Autodesk Inventor part; units mm, degrees
ref_plane "YZ Plane" through (0, 0, 0) normal (1, 0, 0) x (0, 1, 0)
ref_plane "XZ Plane" through (0, 0, 0) normal (0, 1, 0) x (-1, 0, 0)
ref_plane "XY Plane" through (0, 0, 0) normal (0, 0, 1) x (1, 0, 0)
sketch "Sketch1" plane through (0, 0, 0) normal (0, 0, 1) x (1, 0, 0)
  circle A0 centre (0, 0) radius 4
  dimension "d0" = 8
extrude "Extrusion1" add sketch "Sketch1" along normal blind 15
sketch "Sketch2" plane through (0, 0, 15) normal (0, 0, 1) x (1, 0, 0)
  circle A0 centre (0, 0) radius 4
  line L0 (0, -5.6) -> (0, 5.6)
  line L1 (1.5, -3.7081) -> (1.5, 3.7081)
  line L2 (-1.5, -3.7081) -> (-1.5, 3.7081)
  circle A1 centre (0, 0) radius 4
  dimension "d5" = 3
  dimension "d6" = 1.5
extrude "Extrusion2" cut sketch "Sketch2" against normal blind 3 contours L1 A0 L0 | L0 A0 L2
fillet "Fillet1" radius 0.5 14 edges at (-1.5, 0, 15) (1.5, 0, 15) (-1.5, 0, 12) (1.5, 0, 12) (3.3166, -2.2361, 15) (3.3166, 2.2361, 15) (-4, 0, 15) (-1.5, -3.7081, 13.5) (-1.5, 3.7081, 13.5) (1.5, -3.7081, 13.5) (1.5, 3.7081, 13.5) (0, -4, 12) (0, 4, 12) (-4, 0, 0)
properties part number "Locating Pin"
For this review, take the finished solid that the model builds, in its own axes (mm). A direction names the side the tool comes from. Round coordinates to 2 decimals unless told otherwise and drop trailing zeros. Write each loop counter-clockwise with the first axis right and the second up, starting at its lowest first coordinate (ties: lowest second). Pieces come first, ordered by that corner, then holes. Notation, with made-up numbers: M 3.5,-10.5 L 25.5,-10.5 A35 cw 25.5,24.5 Z; hole C 37.25,17 d6. An arc over 180 degrees is marked long. Write item = value, one per line. Start each with the question number.
(1) Clearance check with flat-ended pins moving along their axes: pin 1 Ø0.6 at (x, y) = (0, 1.5) entering from +Z; pin 2 Ø1.5 at (y, z) = (1.5, 11) entering from -X; pin 3 Ø1.5 at (y, z) = (3, 5) entering from -X. State where each tip first meets the part, or that it passes through.
(2) We need section A-A (z = 13). Give the boundary of the cut face in (x, y), then the cut area to 3 significant figures.
(3) The part is to be moulded in two halves that separate along X. For faces 1 (the face through (0, 0, 12)), 2 (the face through (-4, 0, 7)), 3 (the face through (0, 0, 0)), say which applies: +X half, -X half, draft (parallel to the pull), parting line (faces both ways), or undercut.
(4) For faces 4 (the face through (-3, 0, 15)), 5 (the face through (1.5, 0, 14)), list the 3-axis set-ups (+Z, -Z, +X, -X, +Y, -Y) from which the entire face can be reached by the end or side of a thin tool; tool diameter is ignored.
(5) We need section D-D (z = 6.25). Give the boundary of the cut face in (x, y).
(6) We need section B-B (x = 0). Give the boundary of the cut face in (y, z).
(7) For line 1 along Z through (x, y) = (0, 1.25); line 2 along Z through (x, y) = (3.5, 0.5); line 3 along Y through (x, z) = (2.75, 1.25), list the stretches that pass through material, from the lowest coordinate up.
(8) We need section C-C (y = 0). Give the boundary of the cut face in (x, z), then the cut area to 3 significant figures.
Results found:
q1.pin_1 = 12
q1.pin_2 = -3.93
q1.pin_3 = -3.31
q2.outline = M -2.29,-3.28 A0.5 ccw -1.5,-2.87 L -1.5,2.87 A0.5 ccw -2.29,3.28 A4 ccw Z; M 1.5,-2.87 A0.5 ccw 2.29,-3.28 A4 ccw 2.29,3.28 A0.5 ccw 1.5,2.87 Z
q2.area = 26.1 mm²
q3.face_1 = undercut
q3.face_2 = parting line
q3.face_3 = draft
q4.face_4 = +Z, +X, -X, +Y, -Y
q4.face_5 = +Z, +Y, -Y
q5.outline = C 0,0 d8
q6.outline = M -4,0.5 A0.5 ccw -3.5,0 L 3.5,0 A0.5 ccw 4,0.5 L 4,11.5 A0.5 ccw 3.5,12 L -3.5,12 A0.5 ccw -4,11.5 Z
q7.line_1 = 0 to 12
q7.line_2 = 0 to 15
q7.line_3 = -2.9 to 2.9
q8.outline = M -4,0.5 A0.5 ccw -3.5,0 L 3.5,0 A0.5 ccw 4,0.5 L 4,14.5 A0.5 ccw 3.5,15 L 2,15 A0.5 ccw 1.5,14.5 L 1.5,12.5 A0.5 cw 1,12 L -1,12 A0.5 cw -1.5,12.5 L -1.5,14.5 A0.5 ccw -2,15 L -3.5,15 A0.5 ccw -4,14.5 Z
q8.area = 111 mm²
